from build123d import *

# Parameters (mm, degrees)
SKETCH1_W           = 193.294
SKETCH1_H           = 180
BOSS_EXTRUDE1_DEPTH = 3.175
SKETCH2_R           = 2.159
CUT_EXTRUDE1_DEPTH  = 4.175
SKETCH3_R           = 2.159
SKETCH3_R_2         = 2.415341229
CUT_EXTRUDE2_DEPTH  = 4.175
SKETCH4_W           = 21.330448395
SKETCH4_H           = 54.500274109
CUT_EXTRUDE3_DEPTH  = 4.175


with BuildPart() as part:
    # Sketch1 → Boss-Extrude1 (new body)
    with BuildSketch(Plane(origin=(0, 0, 0), x_dir=(1, 0, 0), z_dir=(0, 1, 0))):
        Rectangle(SKETCH1_W, SKETCH1_H)
    extrude(amount=BOSS_EXTRUDE1_DEPTH)

    # Sketch2 → Cut-Extrude1 (cut, through all)
    with BuildSketch(Plane(origin=(0, 3.175, 0), x_dir=(1, 0, 0), z_dir=(0, 1, 0))):
        with Locations((-86.233, 79.586)):
            Circle(SKETCH2_R)
        with Locations((86.233, 79.586)):
            Circle(SKETCH2_R)
        with Locations((86.233, 41.232)):
            Circle(SKETCH2_R)
        with Locations((86.233, 2.878)):
            Circle(SKETCH2_R)
        with Locations((86.233, -35.476)):
            Circle(SKETCH2_R)
        with Locations((-86.233, 41.232)):
            Circle(SKETCH2_R)
        with Locations((-86.233, 2.878)):
            Circle(SKETCH2_R)
        with Locations((-86.233, -35.476)):
            Circle(SKETCH2_R)
        with Locations((-86.233, -73.83)):
            Circle(SKETCH2_R)
        with Locations((86.233, -73.83)):
            Circle(SKETCH2_R)
    extrude(amount=-CUT_EXTRUDE1_DEPTH, mode=Mode.SUBTRACT)

    # Sketch3 → Cut-Extrude2 (cut, through all)
    with BuildSketch(Plane(origin=(0, 3.175, 0), x_dir=(1, 0, 0), z_dir=(0, 1, 0))):
        with Locations((-14.76439348, 7.002233071)):
            Circle(SKETCH3_R)
        with Locations((20.03360652, 7.002233071)):
            Circle(SKETCH3_R)
        with Locations((20.03360652, -77.3)):
            Circle(SKETCH3_R)
        with Locations((-14.76439348, -77.3)):
            Circle(SKETCH3_R)
        with Locations((2.60360652, 85.080051335)):
            Circle(SKETCH3_R_2)
    extrude(amount=-CUT_EXTRUDE2_DEPTH, mode=Mode.SUBTRACT)

    # Sketch4 → Cut-Extrude3 (cut, through all)
    with BuildSketch(Plane(origin=(0, 3.175, 0), x_dir=(1, 0, 0), z_dir=(0, 1, 0))):
        with Locations((1.186420924, 53.941345115)):
            Rectangle(SKETCH4_W, SKETCH4_H)
    extrude(amount=-CUT_EXTRUDE3_DEPTH, mode=Mode.SUBTRACT)


solid = part.part
Can you work these out from the model? Positions are in its coordinate system, mm. Coordinates: 2 decimals unless noted, no trailing zeros. Write each loop counter-clockwise with the first axis right and the second up, starting at its lowest first coordinate (ties: lowest second). Pieces come first, ordered by that corner, then holes.
Q1. Imagine slicing it at B-B, the plane y = 2.05. Count the separate pieces of the cut face and the enclosed holes in it, plus the area to 3 significant figures.
Results found:
separate pieces: 1
enclosed holes: 16
area: 33,400 mm2
Q2. If we mould it in two halves opening along X, with no side actions, what happens to faces 1 (the face through (-1, 3.175, -1)), 2 (the face through (84.076, 1.61, -2.973))? For each: +X half, -X half, draft (parallel to the pull), parting line (faces both ways), or undercut.
Results found:
face 1: draft
face 2: undercut
Q3. Please list where these lines run through material, in increasing order: L1, parallel to X at y = 1.1, z = 77.3; L2, parallel to X at y = 3, z = -32.5; L3, parallel to X at y = 1.5, z = -78.5.
Results found:
L1: x = -96.65 to -16.92, -12.61 to 17.87, 22.19 to 96.65
L2: x = -96.65 to -9.48, 11.85 to 96.65
L3: x = -96.65 to -88.1, -84.37 to -9.48, 11.85 to 84.37, 88.1 to 96.65
Q4. Imagine slicing it at A-A, the plane z = -57. List the corners of the cut face in (x, y) for me (3 decimals).
Results found:
outline: (-96.647, 0) - (-9.479, 0) - (-9.479, 3.175) - (-96.647, 3.175) - close; (11.852, 0) - (96.647, 0) - (96.647, 3.175) - (11.852, 3.175) - close
Q5. For P1, Ø4, axis at x = -86.233, z = 73.83, coming from the +Y side, with a flat end and sliding along its axis, tell me the tip position at first contact or that it passes through.
Results found:
P1: passes through
